```python
from build123d import *

# Parameters (mm, degrees)
ESQUISSE1_W             = 20
ESQUISSE1_H             = 30
BOSS_EXTRU_1_DEPTH      = 10
ESQUISSE2_R             = 6
BOSS_EXTRU_2_DEPTH      = 40
ESQUISSE3_W             = 40
ESQUISSE3_H             = 30
BOSS_EXTRU_3_DEPTH      = 15
ESQUISSE4_R             = 4.5
ENL_V_MAT_EXTRU_1_DEPTH = 55
ENL_V_MAT_EXTRU_3_DEPTH = 55
ESQUISSE8_W             = 40.266643215
ESQUISSE8_H             = 36.212285802
ENL_V_MAT_EXTRU_4_DEPTH = 55


with BuildPart() as part:
    # Esquisse1 → Boss.-Extru.1 (new body)
    with BuildSketch(Plane.XY):
        with Locations((-10, 15)):
            Rectangle(ESQUISSE1_W, ESQUISSE1_H)
    extrude(amount=BOSS_EXTRU_1_DEPTH)

    # Esquisse2 → Boss.-Extru.2 (add)
    with BuildSketch(Plane.XY.offset(10)):
        with Locations((-10, 18)):
            Circle(ESQUISSE2_R)
    extrude(amount=BOSS_EXTRU_2_DEPTH)

    # Esquisse3 → Boss.-Extru.3 (add)
    with BuildSketch(Plane.XZ):
        with Locations((-10, 15)):
            Rectangle(ESQUISSE3_W, ESQUISSE3_H)
    extrude(amount=BOSS_EXTRU_3_DEPTH)

    # Esquisse4 → Enlèv. mat.-Extru.1 (cut)
    with BuildSketch(Plane(origin=(0, 0, 0), x_dir=(-1, 0, 0), z_dir=(0, 0, -1))):
        with Locations((10, -15)):
            Circle(ESQUISSE4_R)
    extrude(amount=-ENL_V_MAT_EXTRU_1_DEPTH, mode=Mode.SUBTRACT)

    # Esquisse5 → Enlèv. mat.-Extru.3 (cut)
    with BuildSketch(Plane(origin=(0, 0, 0), x_dir=(-1, 0, 0), z_dir=(0, 0, -1))):
        with BuildLine():
            Line((30, 0), (25, 0))
            ThreePointArc((25, 0), (28.535533906, -1.464466094), (30, -5))
            Line((30, -5), (30, 0))
        make_face()
        with BuildLine():
            Line((-10, 0), (-10, -5))
            ThreePointArc((-10, -5), (-8.535533906, -1.464466094), (-5, 0))
            Line((-5, 0), (-10, 0))
        make_face()
    extrude(amount=-ENL_V_MAT_EXTRU_3_DEPTH, mode=Mode.SUBTRACT)

    # Esquisse8 → Enlèv. mat.-Extru.4 (cut)
    with BuildSketch(Plane(origin=(0, 0, 0), x_dir=(-1, 0, 0), z_dir=(0, 0, -1))):
        with Locations((10.133321608, 13.106142901)):
            Rectangle(ESQUISSE8_W, ESQUISSE8_H)
    extrude(amount=-ENL_V_MAT_EXTRU_4_DEPTH, mode=Mode.SUBTRACT)


solid = part.part
```
Input: part model. Units: mm. Frame: model coordinates. Coordinates: 2 decimals unless noted, no trailing zeros. Loops run counter-clockwise (first coordinate to the right, second up) from the corner with the lowest first, then second, coordinate; pieces in that order, holes last. Notation, with made-up numbers: (26, 79) -> (68, 79) arc R30 ccw to (68, 110) -> close; hole circle Ø10 at (88.5, 7). An arc over 180 degrees is marked (long way). Use a Markdown table: item, result.
1) Material intervals for line 1 along X through (y, z) = (-14.25, 3.75); line 2 along X through (y, z) = (-12.5, 26.75), sorted ascending. Write a range as from..to.
Results found:
| item | result |
|---|---|
| line 1 | x = -30..-14.44, -5.56..10 |
| line 2 | x = -30..-13.74, -6.26..10 |
2) Cut plane A-A (y = -13.5). Return the cut outline in (x, z), then the cut area to 3 significant figures.
Results found:
| item | result |
|---|---|
| outline | (-30, 0) -> (-14.24, 0) -> (-14.24, 30) -> (-30, 30) -> close; (-5.76, 0) -> (10, 0) -> (10, 30) -> (-5.76, 30) -> close |
| area | 945 mm2 |
3) Cut plane D-D (x = -10). Return the cut outline in (y, z), then the cut area to 3 significant figures.
Results found:
| item | result |
|---|---|
| outline | (-10.5, 0) -> (-5, 0) -> (-5, 30) -> (-10.5, 30) -> close |
| area | 165 mm2 |
4) Cut plane B-B (z = 27.5). Return the cut outline in (x, y), then the cut area to 3 significant figures.
Results found:
| item | result |
|---|---|
| outline | (-30, -15) -> (-14.5, -15) arc R4.5 cw to (-5.5, -15) -> (10, -15) -> (10, -5) -> (-30, -5) -> close |
| area | 368 mm2 |
5) Pull-direction query (X, two-part tool) for faces 1 (the flat face through (10, -10, 15)), 2 (the flat face through (-30, -10, 15)), 3 (the flat face through (-10, -10, 0)), 4 (the cylindrical face through (-10.1, -10.5, 14.8)); classes: released by +X, released by -X, zero draft, split by the parting line, or undercut.
Results found:
| item | result |
|---|---|
| face 1 | released by +X |
| face 2 | released by -X |
| face 3 | zero draft |
| face 4 | undercut |
6) Cut plane C-C (y = -11.5). Return the cut outline in (x, z).
Results found:
| item | result |
|---|---|
| outline | (-30, 0) -> (-12.83, 0) -> (-12.83, 30) -> (-30, 30) -> close; (-7.17, 0) -> (10, 0) -> (10, 30) -> (-7.17, 30) -> close |
